Input: part model. Units: mm. Frame: model coordinates. A direction names the side the tool comes from. Give positions to 0.01 mm unless a question says otherwise; leave off trailing zeros. Write each loop counter-clockwise with the first axis right and the second up, starting at its lowest first coordinate (ties: lowest second). Pieces come first, ordered by that corner, then holes. Notation, with made-up numbers: (-25, 29) - (25, 29) arc R34 ccw to (25, 62) - close; hole circle Ø5 at (72, -37.5). An arc over 180 degrees is marked (long way). Answer as a JSON object with one key per item and string values. Group by question number.
from build123d import *

# Parameters (mm, degrees)
F1_DEPTH = 19.05
F3_DEPTH = 17.78


with BuildPart() as f1:
    # F0 (on Top) → F1 (new body)
    with BuildSketch(Plane.XY):
        with BuildLine():
            Line((59.698993, 65.978541), (-54.601007, 65.978541))
            ThreePointArc((-54.601007, 65.978541), (-56.846071, 65.048605), (-57.776007, 62.803541))
            Line((-57.776007, 62.803541), (-57.776007, -51.496459))
            ThreePointArc((-57.776007, -51.496459), (-56.846071, -53.741523), (-54.601007, -54.671459))
            Line((-54.601007, -54.671459), (-48.251007, -54.671459))
            ThreePointArc((-48.251007, -54.671459), (-46.005943, -55.601395), (-45.076007, -57.846459))
            Line((-45.076007, -57.846459), (-45.076007, -73.721459))
            Line((-45.076007, -73.721459), (-38.726007, -73.721459))
            Line((-38.726007, -73.721459), (-38.726007, -57.846459))
            ThreePointArc((-38.726007, -57.846459), (-37.796071, -55.601395), (-35.551007, -54.671459))
            Line((-35.551007, -54.671459), (40.648993, -54.671459))
            ThreePointArc((40.648993, -54.671459), (42.894057, -55.601395), (43.823993, -57.846459))
            Line((43.823993, -57.846459), (43.823993, -73.721459))
            Line((43.823993, -73.721459), (50.173993, -73.721459))
            Line((50.173993, -73.721459), (50.173993, -57.846459))
            ThreePointArc((50.173993, -57.846459), (51.103929, -55.601395), (53.348993, -54.671459))
            Line((53.348993, -54.671459), (59.698993, -54.671459))
            ThreePointArc((59.698993, -54.671459), (61.944057, -53.741523), (62.873993, -51.496459))
            Line((62.873993, -51.496459), (62.873993, 62.803541))
            ThreePointArc((62.873993, 62.803541), (61.944057, 65.048605), (59.698993, 65.978541))
        make_face()
    extrude(amount=F1_DEPTH)

    # F2 (on face) → F3 (cut)
    with BuildSketch(Plane.XY.offset(19.05)):
        with BuildLine():
            Line((-6.976007, 62.803541), (-53.013507, 62.803541))
            ThreePointArc((-53.013507, 62.803541), (-55.258571, 61.873605), (-56.188507, 59.628541))
            Line((-56.188507, 59.628541), (-56.188507, 40.578541))
            ThreePointArc((-56.188507, 40.578541), (-55.258571, 38.333477), (-53.013507, 37.403541))
            Line((-53.013507, 37.403541), (-49.838507, 37.403541))
            Line((-49.838507, 37.403541), (-49.838507, 31.053541))
            Line((-49.838507, 31.053541), (-53.013507, 31.053541))
            ThreePointArc((-53.013507, 31.053541), (-55.258571, 30.123605), (-56.188507, 27.878541))
            Line((-56.188507, 27.878541), (-56.188507, -16.571459))
            ThreePointArc((-56.188507, -16.571459), (-55.258571, -18.816523), (-53.013507, -19.746459))
            Line((-53.013507, -19.746459), (-49.838507, -19.746459))
            Line((-49.838507, -19.746459), (-49.838507, -26.096459))
            Line((-49.838507, -26.096459), (-53.013507, -26.096459))
            ThreePointArc((-53.013507, -26.096459), (-55.258571, -27.026395), (-56.188507, -29.271459))
            Line((-56.188507, -29.271459), (-56.188507, -48.321459))
            ThreePointArc((-56.188507, -48.321459), (-55.258571, -50.566523), (-53.013507, -51.496459))
            Line((-53.013507, -51.496459), (-3.801007, -51.496459))
            ThreePointArc((-3.801007, -51.496459), (-1.555943, -50.566523), (-0.626007, -48.321459))
            Line((-0.626007, -48.321459), (-0.626007, -45.146459))
            Line((-0.626007, -45.146459), (5.723993, -45.146459))
            Line((5.723993, -45.146459), (5.723993, -48.321459))
            ThreePointArc((5.723993, -48.321459), (6.653929, -50.566523), (8.898993, -51.496459))
            Line((8.898993, -51.496459), (58.111493, -51.496459))
            ThreePointArc((58.111493, -51.496459), (60.356557, -50.566523), (61.286493, -48.321459))
            Line((61.286493, -48.321459), (61.286493, -29.271459))
            ThreePointArc((61.286493, -29.271459), (60.356557, -27.026395), (58.111493, -26.096459))
            Line((58.111493, -26.096459), (54.936493, -26.096459))
            Line((54.936493, -26.096459), (54.936493, -19.746459))
            Line((54.936493, -19.746459), (58.111493, -19.746459))
            ThreePointArc((58.111493, -19.746459), (60.356557, -18.816523), (61.286493, -16.571459))
            Line((61.286493, -16.571459), (61.286493, 27.878541))
            ThreePointArc((61.286493, 27.878541), (60.356557, 30.123605), (58.111493, 31.053541))
            Line((58.111493, 31.053541), (54.936493, 31.053541))
            Line((54.936493, 31.053541), (54.936493, 37.403541))
            Line((54.936493, 37.403541), (58.111493, 37.403541))
            ThreePointArc((58.111493, 37.403541), (60.356557, 38.333477), (61.286493, 40.578541))
            Line((61.286493, 40.578541), (61.286493, 59.628541))
            ThreePointArc((61.286493, 59.628541), (60.356557, 61.873605), (58.111493, 62.803541))
            Line((58.111493, 62.803541), (5.723993, 62.803541))
            ThreePointArc((5.723993, 62.803541), (3.478929, 61.873605), (2.548993, 59.628541))
            Line((2.548993, 59.628541), (2.548993, 56.453541))
            Line((2.548993, 56.453541), (-3.801007, 56.453541))
            Line((-3.801007, 56.453541), (-3.801007, 59.628541))
            ThreePointArc((-3.801007, 59.628541), (-4.730943, 61.873605), (-6.976007, 62.803541))
        make_face()
    extrude(amount=-F3_DEPTH, mode=Mode.SUBTRACT)


solid = f1.part
1) Cut plane B-B on x = 46.5. Return the cut outline in (y, z), and give its area (3 significant figures).
2) Pin query (flat end, axial travel): P1, Ø8, axis at y = -65.5, z = 12.5, coming from the +X side; P2, Ø5, axis at x = -1, z = 9, coming from the -Y side; P3, Ø1, axis at x = 25, y = -40.5, coming from the +Z side. Return the tip coordinate at first contact, or that it passes through.
3) Cut plane A-A on y = -64.5. Return the cut outline in (x, z), and give its area (3 significant figures).
4) Line query: line 1 along X through (y, z) = (57, 16); line 2 along Y through (x, z) = (-32.5, 12.25); line 3 along X through (y, z) = (43.5, 10.25). Output: solid intervals per line, ascending. Write a range as from..to.
5) Cut plane C-C on y = -4. Return the cut outline in (x, z).
6) Mould query, pull axis Y, two halves, no side actions, for faces 5 (the face through (60.38, 30.1, 10.28)), 6 (the face through (-56.87, -53.72, 9.39)), 7 (the face through (62.874, 5, 9)), 8 (the face through (-55.23, 30.15, 10.28)). Classes: +Y half, -Y half, draft (parallel to the pull), parting line (faces both ways), or undercut.
7) Reachability of faces 1 (the face through (2, -54.671, 9)), 2 (the face through (50.174, -66, 9)), 3 (the face through (-57.776, 6, 9)), 4 (the face through (-1, 56.454, 10)) from +Z, -Z, +X, -X, +Y, -Y: full face, straight path, thin tool, end or side. Return the list, or none.
Filled in:
{
 "1": {"outline": "(-73.72, 0) - (65.98, 0) - (65.98, 19.05) - (62.8, 19.05) - (62.8, 1.27) - (-51.5, 1.27) - (-51.5, 19.05) - (-73.72, 19.05) - close", "area": "629 mm²"},
 "2": {"P1": "stops at x = 50.17", "P2": "stops at y = -54.67", "P3": "stops at z = 1.27"},
 "3": {"outline": "(-45.08, 0) - (-38.73, 0) - (-38.73, 19.05) - (-45.08, 19.05) - close; (43.82, 0) - (50.17, 0) - (50.17, 19.05) - (43.82, 19.05) - close", "area": "242 mm²"},
 "4": {"line 1": "x = -57.78..-56.19, -3.8..2.55, 61.29..62.87", "line 2": "y = -54.67..-51.5, 62.8..65.98", "line 3": "x = -57.78..-56.19, 61.29..62.87"},
 "5": {"outline": "(-57.78, 0) - (62.87, 0) - (62.87, 19.05) - (61.29, 19.05) - (61.29, 1.27) - (-56.19, 1.27) - (-56.19, 19.05) - (-57.78, 19.05) - close"},
 "6": {"face 5": "undercut", "face 6": "-Y half", "face 7": "draft", "face 8": "undercut"},
 "7": {"face 1": "+Z, -Z, -Y", "face 2": "+Z, -Z, +X, -Y", "face 3": "+Z, -Z, -X, +Y, -Y", "face 4": "+Z"}
}
